Source: CAD feature listing. Evaluate the final solid. Frame: model axes, mm. Face numbers are marked on the shaded views. A direction names the side the tool comes from. Round coordinates to 2 decimals unless told otherwise and drop trailing zeros. Loops run counter-clockwise (first coordinate to the right, second up) from the corner with the lowest first, then second, coordinate; pieces in that order, holes last. Notation, with made-up numbers: (54.25, 0) -> (81.25, 0) arc R21 cw to (81.25, 20) -> close; hole circle Ø3 at (-9, 68). An arc over 180 degrees is marked (long way). Write item = value, one per line.
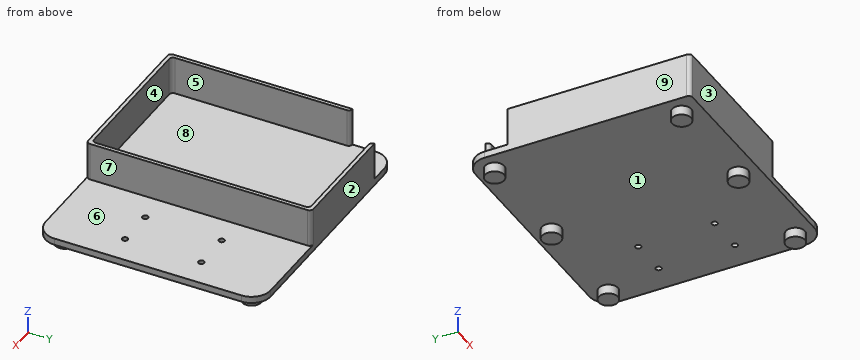
from build123d import *

# Parameters (mm, degrees)
SKETCH_1_W                                 = 50
SKETCH_1_H                                 = 118
EXTRUDE_1_DEPTH                            = 3.5
SKETCH_3_R                                 = 1.5
CUT_EXTRUDE_1_DEPTH                        = 65.1735927
MIRROR_1_AT_THE_SECOND_PLANE_COPY_1_SKET_R = 1.5
MIRROR_1_AT_THE_SECOND_PLANE_COPY_1_DEPTH  = 65.1735927
SKETCH_4_W                                 = 3.5
SKETCH_4_H                                 = 118
EXTRUDE_2_DEPTH                            = 82
EXTRUDE_4_OUTLINE_W                        = 82
EXTRUDE_4_OUTLINE_H                        = 118
EXTRUDE_4_OUTLINE_W_2                      = 78
EXTRUDE_4_OUTLINE_H_2                      = 114
EXTRUDE_4_DEPTH                            = 20
SKETCH_6_W                                 = 2
SKETCH_6_H                                 = 20
SKETCH_6_W_2                               = 18
CUT_EXTRUDE_2_DEPTH                        = 20
SKETCH_7_W                                 = 18
SKETCH_7_H                                 = 20
SKETCH_7_W_2                               = 2
CUT_EXTRUDE_3_DEPTH                        = 20
FILLET_1_R                                 = 10
FILLET_2_R                                 = 2
FILLET_3_R                                 = 2
SKETCH_8_R                                 = 5
EXTRUDE_3_DEPTH                            = 5
SKETCH_9_R                                 = 5
EXTRUDE_4_2_DEPTH                          = 5


# Read off the part's stored shape, not the designer's step: 拉伸-薄壁4
with BuildPart() as part:
    # 草图1 → 凸台-拉伸1 (new body)
    with BuildSketch(Plane.XY):
        Rectangle(SKETCH_1_W, SKETCH_1_H)
    extrude(amount=EXTRUDE_1_DEPTH)

    # 草图3 → 切除-拉伸1 (cut, through all)
    with BuildSketch(Plane.XY.offset(3.5)):
        with Locations((-10, 20)):
            Circle(SKETCH_3_R)
    cut_extrude_1 = extrude(amount=-CUT_EXTRUDE_1_DEPTH, mode=Mode.SUBTRACT)

    # 镜向1: 切除-拉伸1 across plane
    add(cut_extrude_1.mirror(Plane(origin=(0, 0, 0), x_dir=(0, 0, 1), z_dir=(1, 0, 0))), mode=Mode.SUBTRACT)

    # 镜向1 at the second plane: 切除-拉伸1 across plane
    add(cut_extrude_1.mirror(Plane.ZX), mode=Mode.SUBTRACT)

    # 镜向1 at the second plane copy 1 sket → 镜向1 at the second plane copy 1 (cut, through all)
    with BuildSketch(Plane(origin=(0, 0, 3.5), x_dir=(-1, 0, 0), z_dir=(0, 0, 1))):
        with Locations((-10, 20)):
            Circle(MIRROR_1_AT_THE_SECOND_PLANE_COPY_1_SKET_R)
    extrude(amount=-MIRROR_1_AT_THE_SECOND_PLANE_COPY_1_DEPTH, mode=Mode.SUBTRACT)

    # 草图4 → 凸台-拉伸2 (add)
    with BuildSketch(Plane.ZY.offset(25)):
        with Locations((1.75, 0)):
            Rectangle(SKETCH_4_W, SKETCH_4_H)
    extrude(amount=EXTRUDE_2_DEPTH)

    # Extrude 4 outline → Extrude 4 (add)
    with BuildSketch(Plane.XY.offset(3.5)):
        with Locations((-66, 0)):
            Rectangle(EXTRUDE_4_OUTLINE_W, EXTRUDE_4_OUTLINE_H)
        with Locations((-66, 0)):
            Rectangle(EXTRUDE_4_OUTLINE_W_2, EXTRUDE_4_OUTLINE_H_2, mode=Mode.SUBTRACT)
    extrude(amount=EXTRUDE_4_DEPTH)

    # 草图6 → 切除-拉伸2 (cut)
    with BuildSketch(Plane.XZ.offset(-57)):
        with Locations((-106, 13.5)):
            Rectangle(SKETCH_6_W, SKETCH_6_H)
        with Locations((-96, 13.5)):
            Rectangle(SKETCH_6_W_2, SKETCH_6_H)
    extrude(amount=CUT_EXTRUDE_2_DEPTH, mode=Mode.SUBTRACT)

    # 草图7 → 切除-拉伸3 (cut)
    with BuildSketch(Plane.XZ.offset(-57)):
        with Locations((-96, 13.5)):
            Rectangle(SKETCH_7_W, SKETCH_7_H)
        with Locations((-106, 13.5)):
            Rectangle(SKETCH_7_W_2, SKETCH_7_H)
    extrude(amount=-CUT_EXTRUDE_3_DEPTH, mode=Mode.SUBTRACT)

    # 圆角1
    fillet_1_edges = [part.edges().sort_by_distance(p)[0] for p in [
        (25, -59, 1.75),
        (25, 59, 1.75),
        (-107, 59, 1.75),
    ]]
    fillet(fillet_1_edges, radius=FILLET_1_R)

    # 圆角2
    fillet_2_edges = [part.edges().sort_by_distance(p)[0] for p in [
        (-87, 57, 13.5),
        (-107, -59, 11.75),
        (-25, -59, 13.5),
        (-25, 59, 13.5),
        (-105, 37, 13.5),
    ]]
    fillet(fillet_2_edges, radius=FILLET_2_R - 0.0001)  # a hair under: the kernel refuses the full size

    # 圆角3
    fillet_3_edges = [part.edges().sort_by_distance(p)[0] for p in [
        (-27, 57, 13.5),
        (-105, -57, 13.5),
        (-27, -57, 13.5),
    ]]
    fillet(fillet_3_edges, radius=FILLET_3_R)

    # 草图8 → 凸台-拉伸3 (add)
    with BuildSketch(Plane(origin=(0, 0, 0), x_dir=(-1, 0, 0), z_dir=(0, 0, -1))):
        with Locations(Location((-15, 49, 0), (0, 0, 180))):
            Circle(SKETCH_8_R)
        with Locations(Location((97, 49, 0), (0, 0, 180))):
            Circle(SKETCH_8_R)
        with Locations(Location((-15, -49, 0), (0, 0, 180))):
            Circle(SKETCH_8_R)
        with Locations(Location((97, -49, 0), (0, 0, 180))):
            Circle(SKETCH_8_R)
    extrude(amount=EXTRUDE_3_DEPTH)

    # 草图9 → Extrude 4 2 (add)
    with BuildSketch(Plane(origin=(0, 0, 0), x_dir=(-1, 0, 0), z_dir=(0, 0, -1))):
        with Locations(Location((41, 49, 0), (0, 0, 180))):
            Circle(SKETCH_9_R)
        with Locations(Location((41, -49, 0), (0, 0, 180))):
            Circle(SKETCH_9_R)
    extrude(amount=EXTRUDE_4_2_DEPTH)


solid = part.part
1. Section query B-B (y = 20). Return the cut outline in (x, z), then the cut area to 3 significant figures.
Evaluation:
outline = (-107, 0) -> (-11.5, 0) -> (-11.5, 3.5) -> (-25, 3.5) -> (-25, 23.5) -> (-27, 23.5) -> (-27, 3.5) -> (-105, 3.5) -> (-105, 23.5) -> (-107, 23.5) -> close; (-8.5, 0) -> (8.5, 0) -> (8.5, 3.5) -> (-8.5, 3.5) -> close; (11.5, 0) -> (25, 0) -> (25, 3.5) -> (11.5, 3.5) -> close
area = 521 mm²
2. Line query: probe 1 along Y at (x, z) = (10, 1.45); probe 2 along X at (y, z) = (-20, 2.2); probe 3 along Y at (x, z) = (-70, 17.75). Output: solid intervals per line, ascending. Write a range as from..to.
Evaluation:
probe_1 = -59..-21.5, -18.5..18.5, 21.5..59
probe_2 = -107..-11.5, -8.5..8.5, 11.5..25
probe_3 = -59..-57, 57..59
3. Set-up query: the marked faces 1, 2, 3, 4 and 5. Return all of +Z, -Z, +X, -X, +Y, -Y with unobstructed straight access to the full face (end or side cutting, diameter ignored); none if empty.
Evaluation:
face_1 = -Z
face_2 = +Z, -Z, +X, -X, +Y
face_3 = +Z, -Z, +X, -X, -Y
face_4 = +Z
face_5 = +Z, +Y
4. Section query A-A (x = -10). Return the cut outline in (y, z).
Evaluation:
outline = (-59, 0) -> (-21.5, 0) -> (-21.5, 3.5) -> (-59, 3.5) -> close; (-18.5, 0) -> (18.5, 0) -> (18.5, 3.5) -> (-18.5, 3.5) -> close; (21.5, 0) -> (59, 0) -> (59, 3.5) -> (21.5, 3.5) -> close
5. Section query D-D (y = -27). Return the cut outline in (x, z).
Evaluation:
outline = (-107, 0) -> (25, 0) -> (25, 3.5) -> (-25, 3.5) -> (-25, 23.5) -> (-27, 23.5) -> (-27, 3.5) -> (-105, 3.5) -> (-105, 23.5) -> (-107, 23.5) -> close
6. Contact query for flat-ended pins moving along their axis: pin 1 Ø6 at (y, z) = (24.5, 18) entering from +X; pin 2 Ø12 at (x, y) = (-81.5, 11.5) entering from -Z; pin 3 Ø3.5 at (x, y) = (-10, -20) entering from +Z; pin 4 Ø2.5 at (x, y) = (-10, 20) entering from +Z. Output: stop coordinate, or through.
Evaluation:
pin_1 = -25
pin_2 = 0
pin_3 = 3.5
pin_4 = through
7. Mould query, pull axis X, two halves, no side actions, for the marked faces 6, 7, 8 and 9. Classes: released by +X, released by -X, zero draft, split by the parting line, or undercut.
Evaluation:
face_6 = zero draft
face_7 = released by +X
face_8 = undercut
face_9 = released by -X
